Source: CAD feature listing. Evaluate the final solid. Frame: model axes, mm. Coordinates: 2 decimals unless noted, no trailing zeros. Write each loop counter-clockwise with the first axis right and the second up, starting at its lowest first coordinate (ties: lowest second). Pieces come first, ordered by that corner, then holes. Notation, with made-up numbers: (20, 42.25) - (73, 42.25) arc R26 cw to (73, 80.25) - close; hole circle Ø1 at (57, -8). An arc over 180 degrees is marked (long way). One line per item, written item: value.
from build123d import *

# Parameters (mm, degrees)
ESQUISSE4_R = 1.5
ESQUISSE5_W = 1.5
ESQUISSE5_H = 1


with BuildPart() as part:
    # Balayage1: sweep along a path in Esquisse3
    with BuildLine(Plane(origin=(0, 0, 0), x_dir=(-0.5100376925115994, -0.8601520518009844, 0), z_dir=(0.8601520518009843, -0.5100376925115992, 0))) as balayage1_path:
        Line((0, -15), (0, 15))
        Line((0, 15), (191.00019974, 15))
        Line((191.00019974, 15), (191.00019974, -15))
    # Esquisse4 → Balayage1 (sweep)
    with BuildSketch(Plane(origin=(0, 0, 15), x_dir=(-1, 0, 0), z_dir=(0, 0, -1))):
        Circle(ESQUISSE4_R)
    sweep(path=balayage1_path.line, transition=Transition.RIGHT)

    # Esquisse5 → Révolution1 (revolve)
    with BuildSketch(Plane(origin=(0, 0, 0), x_dir=(-0.5100376925115994, -0.8601520518009844, 0), z_dir=(0.8601520518009843, -0.5100376925115992, 0)), mode=Mode.PRIVATE) as r_volution1_sk:
        with Locations((-2.25, -10.5)):
            Rectangle(ESQUISSE5_W, ESQUISSE5_H)
        with Locations((-2.25, 10.5)):
            Rectangle(ESQUISSE5_W, ESQUISSE5_H)
    revolve(r_volution1_sk.sketch.rotate(Axis((0, 0, -11), (0, 0, 1)), 30.666340454), axis=Axis((0, 0, -11), (0, 0, 1)))


solid = part.part
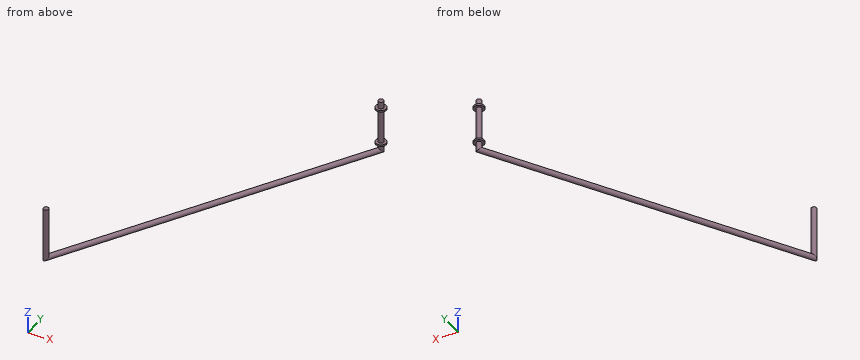
1) Contact query for a flat-ended pin moving along its axis: P1, Ø12, axis at y = -36.5, z = -10, coming from the +X side. Output: stop coordinate, or through.
Values found:
P1: x = -17.62
2) Material intervals for line 1 (Y direction, x = -59, z = -15); line 2 (X direction, y = -127, z = -14), sorted ascending.
Values found:
line 1: -102.44 to -96.56
line 2: -76.61 to -74.01
3) Section query A-A on z = 0.5. Output: boundary loops of the cut face in (x, y), then the cut area to 3 significant figures.
Values found:
outline: circle Ø3 at (-97.42, -164.29); circle Ø3 at (0, 0)
area: 14.1 mm2
